```python
from build123d import *

# Parameters (mm, degrees)
EXTRUDE_1_DEPTH     = 26
EXTRUDE_2_DEPTH     = 19
FILLET_1_R          = 10
SKETCH_5_W          = 161
SKETCH_5_H          = 6
CUT_EXTRUDE_1_DEPTH = 52


with BuildPart() as part:
    # Sketch 1 → Extrude 1 (new body)
    with BuildSketch(Plane.XY):
        Polygon((-168, 0), (168, 0), (183, 0), (183, -340), (168, -340), (168, -20), (-168, -20), (-168, -340), (-183, -340), (-183, 0), align=None)
    extrude(amount=EXTRUDE_1_DEPTH)

    # Sketch 1_4 → Extrude 2 (add)
    with BuildSketch(Plane.XY):
        Polygon((171, 0), (168, 0), (168, -20), (168, -340), (171, -340), align=None)
        Polygon((-168, -20), (-168, 0), (-171, 0), (-171, -340), (-168, -340), align=None)
    extrude(amount=-EXTRUDE_2_DEPTH)

    # Fillet 1
    fillet_1_edges = [part.edges().sort_by_distance(p)[0] for p in [
        (169.5, 0, -19),
        (169.5, -340, -19),
        (-169.5, -340, -19),
        (-169.5, 0, -19),
    ]]
    fillet(fillet_1_edges, radius=FILLET_1_R)

    # Sketch 5 → Cut-Extrude 1 (cut)
    with BuildSketch(Plane(origin=(0, 0, 0), x_dir=(1, 0, 0), z_dir=(0, 1, 0))):
        with Locations((-87.5, -3)):
            Rectangle(SKETCH_5_W, SKETCH_5_H)
        with Locations((87.5, -3)):
            Rectangle(SKETCH_5_W, SKETCH_5_H)
    extrude(amount=-CUT_EXTRUDE_1_DEPTH, mode=Mode.SUBTRACT)


solid = part.part
```
Here's how the part is built. I have some questions about the finished solid (model axes, mm). A direction names the side the tool comes from. Give positions to 0.01 mm unless a question says otherwise; leave off trailing zeros. Loops run counter-clockwise (first coordinate to the right, second up) from the corner with the lowest first, then second, coordinate; pieces in that order, holes last. Notation, with made-up numbers: M 56.25,-19.75 L 81.25,-19.75 A16 ccw 81.25,-6.75 Z; hole C 47,63 d1. An arc over 180 degrees is marked long. Put each result on its own line as item: value. Start each with the question number.
(1) I want a section at D-D on x = 27. Please give me the cut outline in (y, z).
(2) I want a section at A-A on y = -133. Please give me the cut outline in (x, z).
(3) For faces 1 (the flat face through (171, -172, -9)), 2 (the flat face through (86, -10, 6)), 3 (the flat face through (-177, -168, 0)), 4 (the flat face through (2, -20, 16)), which set-ups out of +Z, -Z, +X, -X, +Y, -Y let a thin tool reach every point of the face, with its end or its side?
(4) I want a section at B-B on z = -14.5. Please give me the cut outline in (x, y).
(5) Will these pins go through, and if not, where does the flat tip stop? pin 1 Ø7 at (x, y) = (-1, -9.5) entering from -Z; pin 2 Ø16 at (x, y) = (85.5, -11) entering from -Z; pin 3 Ø15 at (y, z) = (-154.5, -13) entering from -X.
(6) I want a section at C-C on z = 19.5. Please give me the cut outline in (x, y), then the cut area to 3 significant figures.
(7) If we mould it in two halves opening along X, with no side actions, what happens to faces 5 (the flat face through (3, 0, 17)), 6 (the flat face through (-171, -168, -9)), 7 (the flat face through (-168, -172, 4))? For each: +X half, -X half, draft (parallel to the pull), parting line (faces both ways), or undercut.
(8) I need wall thicknesses on line 1 along X through (y, z) = (-279, 15); line 2 along X through (y, z) = (-31, -1.5); line 3 along Y through (x, z) = (83, 16). Which ranges of each line are inside material? Lowest first, please. Write a range as [from, to].
Answer block:
1. outline: M -20,6 L 0,6 L 0,26 L -20,26 Z
2. outline: M -183,0 L -171,0 L -171,-19 L -168,-19 L -168,26 L -183,26 Z; M 168,-19 L 171,-19 L 171,0 L 183,0 L 183,26 L 168,26 Z
3. face 1: -Z, +X, +Y, -Y
3. face 2: -Z, +Y, -Y
3. face 3: -Z, -X, +Y, -Y
3. face 4: +Z, -Z, -Y
4. outline: M -171,-338.35 L -168,-338.35 L -168,-1.65 L -171,-1.65 Z; M 168,-338.35 L 171,-338.35 L 171,-1.65 L 168,-1.65 Z
5. pin 1: z = 0
5. pin 2: z = 6
5. pin 3: x = -171
6. outline: M -183,-340 L -168,-340 L -168,-20 L 168,-20 L 168,-340 L 183,-340 L 183,0 L -183,0 Z
6. area: 16,900 mm^2
7. face 5: draft
7. face 6: -X half
7. face 7: undercut
8. line 1: [-183, -168], [168, 183]
8. line 2: [-171, -168], [168, 171]
8. line 3: [-20, 0]
